```python
from build123d import *

# Parameters (mm, degrees)
SKETCH_1_R      = 13
SKETCH_1_R_2    = 2.5
EXTRUDE_1_DEPTH = 3
CHAMFER_1_SIZE  = 0.2


with BuildPart() as part:
    # 草图1 → 凸台-拉伸1 (new, symmetric)
    with BuildSketch(Plane.XY):
        Circle(SKETCH_1_R)
        Circle(SKETCH_1_R_2, mode=Mode.SUBTRACT)
    extrude(amount=EXTRUDE_1_DEPTH, both=True)

    # 草图2 → 切除-旋转1 (revolve, cut)
    with BuildSketch(Plane(origin=(0, 0, 0), x_dir=(0, 0, -1), z_dir=(1, 0, 0)), mode=Mode.PRIVATE) as cut_revolve_1_sk:
        Polygon((0, 11), (2.301135457, 13), (-2.301135457, 13), align=None)
    revolve(cut_revolve_1_sk.sketch.rotate(Axis((0, 0, 0), (0, 0, -1)), 90), axis=Axis((0, 0, 0), (0, 0, -1)), mode=Mode.SUBTRACT)

    # 倒角1
    chamfer_1_edges = [part.edges().sort_by_distance(p)[0] for p in [
        (-13, 0, -3),
        (-13, 0, 3),
        (-2.5, 0, -3),
        (-2.5, 0, 3),
    ]]
    chamfer(chamfer_1_edges, length=CHAMFER_1_SIZE)


solid = part.part
```
Read the model definition and answer for the solid it produces. Units are mm, in the model's axes. A direction names the side the tool comes from. Round coordinates to 2 decimals unless told otherwise and drop trailing zeros. Write each loop counter-clockwise with the first axis right and the second up, starting at its lowest first coordinate (ties: lowest second). Pieces come first, ordered by that corner, then holes. Notation, with made-up numbers: (79, 46.5) - (116, 46.5) arc R19 cw to (116, 56.5) - close; hole circle Ø10 at (29, -0.75). An arc over 180 degrees is marked (long way). One line per item, written item: value.
Q1. Find section B-B (z = -0.9). Determine the outline of the cut face in (x, y), and give its area (3 significant figures).
The answers:
outline: circle Ø23.56 at (0, 0); hole circle Ø5 at (0, 0)
area: 416 mm2
Q2. Find section A-A (x = 0). Determine the outline of the cut face in (y, z).
The answers:
outline: (-13, -2.8) - (-12.8, -3) - (-2.7, -3) - (-2.5, -2.8) - (-2.5, 2.8) - (-2.7, 3) - (-12.8, 3) - (-13, 2.8) - (-13, 2.3) - (-11, 0) - (-13, -2.3) - close; (2.5, -2.8) - (2.7, -3) - (12.8, -3) - (13, -2.8) - (13, -2.3) - (11, 0) - (13, 2.3) - (13, 2.8) - (12.8, 3) - (2.7, 3) - (2.5, 2.8) - close
Q3. Straight lines are drawn through the part: line 1 (Y direction, x = -1.75, z = -2.1); line 2 (Y direction, x = -2, z = -0.3); line 3 (Z direction, x = 6.25, y = 10.5). For each, find the intervals that lie inside material, in ascending order. Write a range as from..to.
The answers:
line 1: y = -12.71..-1.79, 1.79..12.71
line 2: y = -11.08..-1.5, 1.5..11.08
line 3: z = -3..-1.4, 1.4..3
Q4. Which of the six approach directions +Z, -Z, +X, -X, +Y, -Y give full straight-line access (tool end or side, diameter ignored) to faces 4 (the flat face through (0, 3, 3)), 5 (the conical face through (5.13, 9.87, -0.14))?
The answers:
face 4: +Z, +X, -X, +Y, -Y
face 5: none
Q5. Each of these flat-tipped pins is pushed along its axis until it touches: P1, Ø2, axis at x = 9.5, z = 0.5, coming from the +Y side; P2, Ø1, axis at x = 8, z = -1, coming from the +Y side; P3, Ø3, axis at x = 0.5, z = 0.5, coming from the -Y side. Where does it stop, or does it pass through?
The answers:
P1: stops at y = 8.24
P2: stops at y = 9.48
P3: stops at y = -12.73
Q6. For a pull along X with two mould halves and no side action, classify faces 1 (the cylindrical face through (-10.316, -7.91, -2.547)), 2 (the flat face through (0, 3, -3)), 3 (the cylindrical face through (-0.54, -2.44, -0.04)) as pulls with the +X half, pulls with the -X half, needs draft (parallel to the pull), parting line crosses it, or undercut.
The answers:
face 1: parting line crosses it
face 2: needs draft
face 3: undercut
